Geometry check sheet. Reference: the model listing, model coordinates, mm. Face numbers are marked on the shaded views. A direction names the side the tool comes from. Give positions to 0.01 mm unless a question says otherwise; leave off trailing zeros. Order: outer loops, then holes, each group sorted by start corner. A loop starts at its lowest first (then second) coordinate and runs counter-clockwise, first axis right, second up. Notation, with made-up numbers: M 84,11 L 109,11 A14 cw 109,27 Z; hole C 21.25,-9.5 d10. An arc over 180 degrees is marked long. Answer as a JSON object with one key per item and string values. Group by question number.
from build123d import *

# Parameters (mm, degrees)
SKETCH1_W           = 41
SKETCH1_H           = 118.5
BOSS_EXTRUDE1_DEPTH = 5
SKETCH2_W           = 21
SKETCH2_H           = 10.2
CUT_EXTRUDE1_DEPTH  = 6
SKETCH9_R           = 1.75
CUT_EXTRUDE4_DEPTH  = 6
CUT_EXTRUDE5_DEPTH  = 6
BOSS_EXTRUDE4_DEPTH = 23.9
SKETCH16_W          = 2
SKETCH16_H          = 103.3
BOSS_EXTRUDE5_DEPTH = 23.9
CUT_EXTRUDE8_DEPTH  = 22.5
BOSS_EXTRUDE6_DEPTH = 28.9
SKETCH25_W          = 6.711597152
SKETCH25_H          = 4.45
CUT_EXTRUDE9_DEPTH  = 6
SKETCH26_R          = 1.75
CUT_EXTRUDE10_DEPTH = 119.5


with BuildPart() as part:
    # Sketch1 → Boss-Extrude1 (new body)
    with BuildSketch(Plane(origin=(0, 0, 0), x_dir=(1, 0, 0), z_dir=(0, 1, 0))):
        with Locations((20.5, 59.25)):
            Rectangle(SKETCH1_W, SKETCH1_H)
    extrude(amount=BOSS_EXTRUDE1_DEPTH)

    # Sketch2 → Cut-Extrude1 (cut, through all)
    with BuildSketch(Plane(origin=(0, 5, 0), x_dir=(1, 0, 0), z_dir=(0, 1, 0))):
        with Locations((20.5, 113.4)):
            Rectangle(SKETCH2_W, SKETCH2_H)
    extrude(amount=-CUT_EXTRUDE1_DEPTH, mode=Mode.SUBTRACT)

    # Sketch9 → Cut-Extrude4 (cut, through all)
    with BuildSketch(Plane(origin=(0, 5, 0), x_dir=(1, 0, 0), z_dir=(0, 1, 0))):
        with Locations((5, 113.5)):
            Circle(SKETCH9_R)
        with Locations((36, 113.5)):
            Circle(SKETCH9_R)
    extrude(amount=-CUT_EXTRUDE4_DEPTH, mode=Mode.SUBTRACT)

    # Sketch11 → Cut-Extrude5 (cut, through all)
    with BuildSketch(Plane(origin=(0, 5, 0), x_dir=(1, 0, 0), z_dir=(0, 1, 0))):
        Polygon((15.5, 0), (0, 98.3), (0, 0), align=None)
        Polygon((25.5, 0), (41, 98.3), (41, 0), align=None)
    extrude(amount=-CUT_EXTRUDE5_DEPTH, mode=Mode.SUBTRACT)

    # Sketch12 → Boss-Extrude4 (add)
    with BuildSketch(Plane(origin=(0, 5, 0), x_dir=(1, 0, 0), z_dir=(0, 1, 0))):
        Polygon((25.5, 0), (15.5, 0), (14.711597152, 5), (26.288402848, 5), align=None)
    extrude(amount=BOSS_EXTRUDE4_DEPTH)

    # Sketch16 → Boss-Extrude5 (add)
    with BuildSketch(Plane(origin=(0, 5, 0), x_dir=(1, 0, 0), z_dir=(0, 1, 0))):
        with Locations((20.5, 56.65)):
            Rectangle(SKETCH16_W, SKETCH16_H)
    extrude(amount=BOSS_EXTRUDE5_DEPTH)

    # Sketch17 → Cut-Extrude8 (cut, through all)
    with BuildSketch(Plane.ZY.offset(-19.5)):
        Polygon((-108.4, 5), (-5, 28.9), (-108.3, 28.9), align=None)
    extrude(amount=-CUT_EXTRUDE8_DEPTH, mode=Mode.SUBTRACT)

    # Sketch23 → Boss-Extrude6 (add)
    with BuildSketch(Plane(origin=(0, 28.9, 0), x_dir=(1, 0, 0), z_dir=(0, 1, 0))):
        Polygon((26.288402848, 5), (33, 5), (33, 0), (25.5, 0), align=None)
        Polygon((14.711597152, 5), (8, 5), (8, 0), (15.5, 0), align=None)
    extrude(amount=-BOSS_EXTRUDE6_DEPTH)

    # Sketch25 → Cut-Extrude9 (cut, through all)
    with BuildSketch(Plane(origin=(0, 0, -5), x_dir=(-1, 0, 0), z_dir=(0, 0, -1))):
        with Locations((-11.355798576, 2.225)):
            Rectangle(SKETCH25_W, SKETCH25_H)
        with Locations((-29.644201424, 2.225)):
            Rectangle(SKETCH25_W, SKETCH25_H)
        with Locations((-11.355798576, 26.675)):
            Rectangle(SKETCH25_W, SKETCH25_H)
        with Locations((-29.644201424, 26.675)):
            Rectangle(SKETCH25_W, SKETCH25_H)
    extrude(amount=-CUT_EXTRUDE9_DEPTH, mode=Mode.SUBTRACT)

    # Sketch26 → Cut-Extrude10 (cut, through all)
    with BuildSketch(Plane.XY):
        with Locations((13, 19.45)):
            Circle(SKETCH26_R)
        with Locations((28, 19.45)):
            Circle(SKETCH26_R)
        with Locations((13, 9.45)):
            Circle(SKETCH26_R)
        with Locations((28, 9.45)):
            Circle(SKETCH26_R)
    extrude(amount=-CUT_EXTRUDE10_DEPTH, mode=Mode.SUBTRACT)


solid = part.part
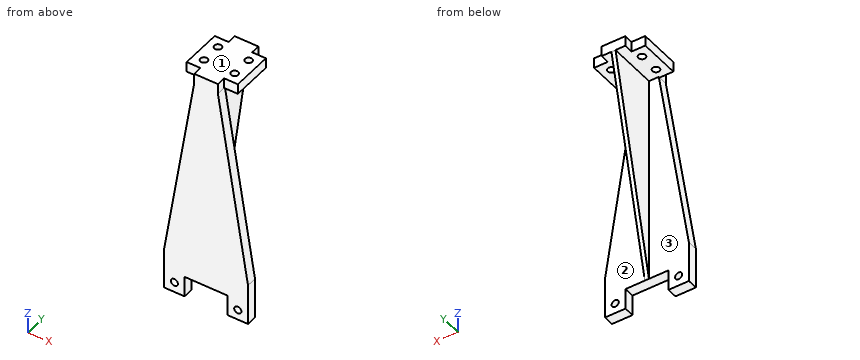
1. Cross-section at D-D (x = 28). Record the cut outline in (y, z), and give its area (3 significant figures).
2. Access from +Z, -Z, +X, -X, +Y, -Y to the whole of each face (thin tool, end or side, straight path). Record for the marked faces 1, 2 and 3.
3. Depth check by flat-ended pin: pin 1 (1.5 mm diameter, centred on x = 10.5, z = -2, fed in from +Y); pin 2 (3.5 mm diameter, centred on y = 3, z = -3.5, fed in from -X); pin 3 (6 mm diameter, centred on x = 27.5, z = -61.5, fed in from +Y). Enter the tip coordinate at first touch or a pass-through.
4. Thickness scan on line 1 along Y through (x, z) = (13, -3.85); line 2 along Y through (x, z) = (19, -35); line 3 along Z through (x, y) = (17.5, 5.25). Record the ranges inside material, lowest first. Write a range as [from, to].
5. Cross-section at A-A (z = -113.5). Record the cut outline in (x, y), and give its area (3 significant figures).
6. Cross-section at B-B (x = 36). Record the cut outline in (y, z), and give its area (3 significant figures).
7. Cross-section at C-C (y = 9.45). Record the cut outline in (x, z).
Report:
{
 "1": {"outline": "M 0,-108.3 L 5,-108.3 L 5,-15.85 L 0,-15.85 Z; M 4.45,-5 L 7.7,-5 L 7.7,0 L 4.45,0 Z; M 11.2,-5 L 17.7,-5 L 17.7,0 L 11.2,0 Z; M 21.2,-5 L 24.45,-5 L 24.45,0 L 21.2,0 Z", "area": "527 mm2"},
 "2": {"face 1": "+Z, +X, -X, +Y, -Y", "face 2": "-Z, +X, +Y", "face 3": "-Z, -X, +Y"},
 "3": {"pin 1": "stops at y = 24.45", "pin 2": "stops at x = 8", "pin 3": "stops at y = 5"},
 "4": {"line 1": "y = [4.45, 7.7], [11.2, 17.7], [21.2, 24.45]", "line 2": "y = [0, 5]", "line 3": "z = [-5, 0]"},
 "5": {"outline": "M 0,0 L 3.25,0 L 3.25,5 L 0,5 Z; M 6.75,0 L 10,0 L 10,5 L 6.75,5 Z; M 31,0 L 34.25,0 L 34.25,5 L 31,5 Z; M 37.75,0 L 41,0 L 41,5 L 37.75,5 Z", "area": "65.0 mm2"},
 "6": {"outline": "M 0,-118.5 L 5,-118.5 L 5,-115.25 L 0,-115.25 Z; M 0,-111.75 L 5,-111.75 L 5,-66.59 L 0,-66.59 Z", "area": "242 mm2"},
 "7": {"outline": "M 8,-5 L 11.25,-5 L 11.25,0 L 8,0 Z; M 14.75,-5 L 19.5,-5 L 19.5,-89.15 L 21.5,-89.15 L 21.5,-5 L 26.25,-5 L 26.25,0 L 14.75,0 Z; M 29.75,-5 L 33,-5 L 33,0 L 29.75,0 Z"}
}
